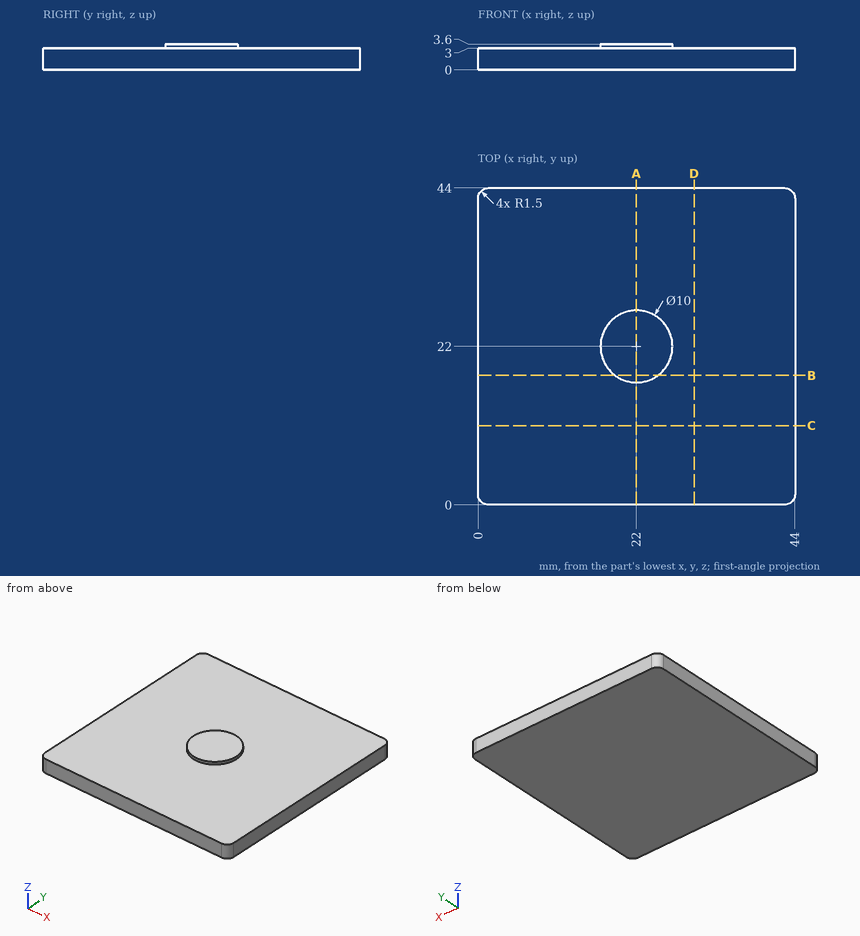
The drawing under review shows one solid part. Ordinate dimensions are in mm from its lowest x, y, z. Coordinates: 2 decimals unless noted, no trailing zeros. Write each loop counter-clockwise with the first axis right and the second up, starting at its lowest first coordinate (ties: lowest second). Pieces come first, ordered by that corner, then holes. Notation, with made-up numbers: M 0,28 L 39,28 A9 ccw 39,45 Z; hole C 89,-27 d2. An arc over 180 degrees is marked long. Answer as a JSON object with one key per item and string values.
Item 1: Add section C-C, the plane y = 11. Give the boundary of the cut face in (x, z).
Outcome:
{"outline": "M 0,0 L 44,0 L 44,3 L 0,3 Z"}
Item 2: Add section A-A, the plane x = 22. Give the boundary of the cut face in (y, z), and give its area (3 significant figures).
Outcome:
{"outline": "M 0,0 L 44,0 L 44,3 L 27,3 L 27,3.6 L 17,3.6 L 17,3 L 0,3 Z", "area": "138 mm²"}
Item 3: Wall thickness on probe 1 along Z at (x, y) = (25.5, 31); probe 2 along Y at (x, z) = (23.5, 3.25); probe 3 along X at (y, z) = (18.5, 3.45): over which ranges is each line inside the solid? List them lowest first.
Outcome:
{"probe 1": "0 to 3", "probe 2": "17.23 to 26.77", "probe 3": "18.43 to 25.57"}
Item 4: Add section B-B, the plane y = 18. Give the boundary of the cut face in (x, z).
Outcome:
{"outline": "M 0,0 L 44,0 L 44,3 L 25,3 L 25,3.6 L 19,3.6 L 19,3 L 0,3 Z"}
